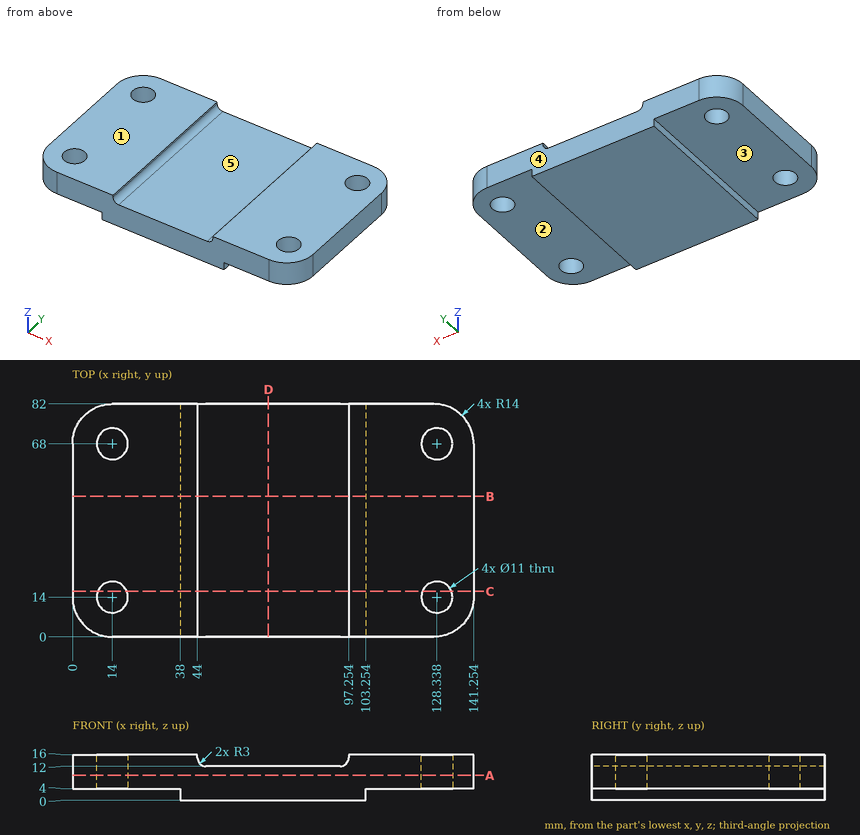
Could you check a few things on this drawing? It's one solid part, dimensions in mm from its lowest x, y, z. A direction names the side the tool comes from. Round coordinates to 2 decimals unless told otherwise and drop trailing zeros. Loops run counter-clockwise (first coordinate to the right, second up) from the corner with the lowest first, then second, coordinate; pieces in that order, holes last.
Q1. I want a section at C-C (y = 16). Write out the boundary of the cut face in (x, z), and give its area (3 significant figures).
Q2. On a 3-axis mill with a long thin cutter (end or side, diameter ignored), from which of +Z, -Z, +X, -X, +Y, -Y can I reach the whole of each face in a straight line? I mean the marked faces 1, 2, 3, 4 and 5. Say none if no direction works.
Q3. I want a section at D-D (x = 69). Write out the boundary of the cut face in (y, z).
Q4. I want a section at B-B (y = 49.5). Write out the boundary of the cut face in (x, z), and give its area (3 significant figures).
Q5. For P1, Ø2, axis at y = 24, z = 1.5, coming from the +X side; P2, Ø4.5, axis at y = 32, z = 1.5, coming from the -X side; P3, Ø1.5, axis at y = 72, z = 6.5, coming from the +X side, each with a flat end and sliding along its axis, tell me the tip position at first contact or that it passes through.
Q6. Please list where these lines run through material, in increasing order: L1, parallel to X at y = 68.5, z = 11.25 (1 decimal); L2, parallel to Y at x = 14, z = 10.25; L3, parallel to Y at x = 18, z = 13 (1 decimal).
Q7. I want a section at A-A (z = 8.75). Write out the boundary of the cut face in (x, y), and give its area (3 significant figures).
Answer below:
1. outline: (0, 4) - (8.88, 4) - (8.88, 16) - (0, 16) - close; (19.12, 4) - (38, 4) - (38, 0) - (103.25, 0) - (103.25, 4) - (123.21, 4) - (123.21, 16) - (97.25, 16) - (97.25, 15) arc R3 cw to (94.25, 12) - (47, 12) arc R3 cw to (44, 15) - (44, 16) - (19.12, 16) - close; (133.46, 4) - (141.25, 4) - (141.25, 16) - (133.46, 16) - close
1. area: 1,500 mm2
2. face 1: +Z, +X, -X, +Y, -Y
2. face 2: -Z, +X, +Y, -Y
2. face 3: -Z, -X, +Y, -Y
2. face 4: +Z, -Z, +X, -X, +Y
2. face 5: +Z, +Y, -Y
3. outline: (0, 0) - (82, 0) - (82, 12) - (0, 12) - close
4. outline: (0, 4) - (38, 4) - (38, 0) - (103.25, 0) - (103.25, 4) - (141.25, 4) - (141.25, 16) - (97.25, 16) - (97.25, 15) arc R3 cw to (94.25, 12) - (47, 12) arc R3 cw to (44, 15) - (44, 16) - (0, 16) - close
4. area: 1,750 mm2
5. P1: stops at x = 103.25
5. P2: stops at x = 38
5. P3: stops at x = 140.87
6. L1: x = 0 to 8.5, 19.5 to 122.9, 133.8 to 141.2
6. L2: y = 0 to 8.5, 19.5 to 62.5, 73.5 to 82
6. L3: y = 0 to 10.2, 17.8 to 64.2, 71.8 to 82
7. outline: (0, 14) arc R14 ccw to (14, 0) - (127.25, 0) arc R14 ccw to (141.25, 14) - (141.25, 68) arc R14 ccw to (127.25, 82) - (14, 82) arc R14 ccw to (0, 68) - close; hole circle Ø11 at (14, 14); hole circle Ø11 at (14, 68); hole circle Ø11 at (128.34, 14); hole circle Ø11 at (128.34, 68)
7. area: 11,000 mm2
